Verification items for the finished model (mm, model axes). A direction names the side the tool comes from. Coordinates: 2 decimals unless noted, no trailing zeros. Loops run counter-clockwise (first coordinate to the right, second up) from the corner with the lowest first, then second, coordinate; pieces in that order, holes last. Notation, with made-up numbers: (52, 22) -> (67, 22) arc R25 ccw to (67, 58) -> close; hole circle Ø7 at (52, -22). An arc over 180 degrees is marked (long way). Write item = value, one per line.
```python
from build123d import *

# Parameters (mm, degrees)
MODEL_R                 = 6
MODEL_R_2               = 8
MODEL_W                 = 32
MODEL_H                 = 32
SALIENTE_EXTRUIR1_DEPTH = 3


with BuildPart() as part:
    # Model → Saliente-Extruir1 (new body)
    with BuildSketch(Plane.XY):
        Polygon((58.7498, 90.00776192), (58.7498, -37.99223808), (45.7498, -37.99223808), (45.7498, -67.99223808), (41.7498, -67.99223808), (39.7498, -62.99223808), (41.7498, -62.99223808), (41.7498, -59.99223808), (25.7498, -59.99223808), (25.7498, -62.99223808), (27.7498, -62.99223808), (25.7498, -67.99223808), (21.7498, -67.99223808), (21.7498, -37.99223808), (8.7498, -37.99223808), (8.7498, 90.00776192), align=None)
        with Locations((33.7498, 55.30776192)):
            Circle(MODEL_R, mode=Mode.SUBTRACT)
        with Locations((20.7498, 74.50776192)):
            Circle(MODEL_R_2, mode=Mode.SUBTRACT)
        with Locations((46.7498, 74.50776192)):
            Circle(MODEL_R_2, mode=Mode.SUBTRACT)
        with Locations((33.7498, 24.30776192)):
            Rectangle(MODEL_W, MODEL_H, mode=Mode.SUBTRACT)
    extrude(amount=SALIENTE_EXTRUIR1_DEPTH)


solid = part.part
```
1) Sectioned sample at A-A, the plane y = 10. Record the cut outline in (x, z).
Ans:
outline = (8.75, 0) -> (17.75, 0) -> (17.75, 3) -> (8.75, 3) -> close; (49.75, 0) -> (58.75, 0) -> (58.75, 3) -> (49.75, 3) -> close
2) Release check for a two-part mould opening along X. For faces 4 (the face through (34, 8.308, 1)), 5 (the face through (44, -67.992, 1)), 6 (the face through (34, 40.308, 1)), 7 (the face through (58.75, 27, 1)) record: pulls with the +X half, pulls with the -X half, needs draft (parallel to the pull), parting line crosses it, or undercut.
Ans:
face_4 = undercut
face_5 = needs draft
face_6 = undercut
face_7 = pulls with the +X half
3) Sectioned sample at D-D, the plane y = 53. Record the cut outline in (x, z), plus the area to 3 significant figures.
Ans:
outline = (8.75, 0) -> (28.21, 0) -> (28.21, 3) -> (8.75, 3) -> close; (39.29, 0) -> (58.75, 0) -> (58.75, 3) -> (39.29, 3) -> close
area = 117 mm2
4) Material ranges on line 1 (Y direction, x = 29.5, z = 1.75); line 2 (Y direction, x = 22.5, z = 0.4); line 3 (X direction, y = 17, z = 0.45), recorded low to high.
Ans:
line_1 = -59.99 to 8.31, 40.31 to 51.07, 59.54 to 90.01
line_2 = -67.99 to 8.31, 40.31 to 66.7, 82.31 to 90.01
line_3 = 8.75 to 17.75, 49.75 to 58.75
5) Sectioned sample at C-C, the plane y = 80.5. Record the cut outline in (x, z).
Ans:
outline = (8.75, 0) -> (15.45, 0) -> (15.45, 3) -> (8.75, 3) -> close; (26.05, 0) -> (41.45, 0) -> (41.45, 3) -> (26.05, 3) -> close; (52.05, 0) -> (58.75, 0) -> (58.75, 3) -> (52.05, 3) -> close
6) Depth check by flat-ended pin: pin 1 Ø0.9 at (x, z) = (32, 1) entering from -Y; pin 2 Ø1.5 at (x, z) = (15, 2) entering from -Y; pin 3 Ø14.5 at (x, y) = (20.75, 74.51) entering from -Z; pin 4 Ø1.5 at (y, z) = (-57, 1) entering from +X. Enter the tip coordinate at first touch or a pass-through.
Ans:
pin_1 = -59.99
pin_2 = -37.99
pin_3 = through
pin_4 = 45.75
7) Sectioned sample at B-B, the plane z = 1. Record the cut outline in (x, y).
Ans:
outline = (8.75, -37.99) -> (21.75, -37.99) -> (21.75, -67.99) -> (25.75, -67.99) -> (27.75, -62.99) -> (25.75, -62.99) -> (25.75, -59.99) -> (41.75, -59.99) -> (41.75, -62.99) -> (39.75, -62.99) -> (41.75, -67.99) -> (45.75, -67.99) -> (45.75, -37.99) -> (58.75, -37.99) -> (58.75, 90.01) -> (8.75, 90.01) -> close; hole circle Ø16 at (20.75, 74.51); hole (17.75, 8.31) -> (49.75, 8.31) -> (49.75, 40.31) -> (17.75, 40.31) -> close; hole circle Ø12 at (33.75, 55.31); hole circle Ø16 at (46.75, 74.51)
8) Tool access check on faces 1 (the face through (15, -37.992, 1)), 2 (the face through (26.764, -65.457, 1.479)), 3 (the face through (49.75, 24, 1)). Record the directions out of +Z, -Z, +X, -X, +Y, -Y that give a thin tool (end or side, any length) a straight path to the whole face; none if there is none.
Ans:
face_1 = +Z, -Z, -X, -Y
face_2 = +Z, -Z, -Y
face_3 = +Z, -Z
